Can you work these out from the model? Positions are in its coordinate system, mm. A direction names the side the tool comes from. Coordinates: 2 decimals unless noted, no trailing zeros. Order: outer loops, then holes, each group sorted by start corner. A loop starts at its lowest first (then second) coordinate and runs counter-clockwise, first axis right, second up. Notation, with made-up numbers: (22.25, 64) -> (43.25, 64) arc R31 cw to (43.25, 98) -> close; hole circle Ø1 at (-12, 39.5). An arc over 180 degrees is marked (long way). Answer in a Markdown table with one row per item.
```python
from build123d import *

# Parameters (mm, degrees)
EXTRUDE_1_DEPTH       = 2.5
SKETCH_1_3_W          = 21.9
SKETCH_1_3_H          = 3
EXTRUDE_2_DEPTH       = 0.5
SKETCH_2_R            = 1
CUT_EXTRUDE_1_DEPTH   = 34.660057049
SKETCH_3_W            = 21.9
SKETCH_3_H            = 3
CUT_EXTRUDE_2_DEPTH   = 1.5
SKETCH_4_W            = 39.2
SKETCH_4_H            = 52.23
EXTRUDE_3_DEPTH       = 1
CUT_EXTRUDE_START     = -1
CUT_EXTRUDE_3_DEPTH   = 1
FILLET_1_R            = 4
CUT_EXTRUDE_1_2_DEPTH = 1


with BuildPart() as part:
    # Sketch 1 → Extrude 1 (new body)
    with BuildSketch(Plane(origin=(0, 0, 0), x_dir=(1, 0, 0), z_dir=(0, 1, 0))):
        with BuildLine():
            ThreePointArc((13.158319986, 21.726795167), (16.799919909, 20.21839509), (18.308319986, 16.576795167))
            Line((18.308319986, 16.576795167), (18.308319986, 26.726795167))
            Line((18.308319986, 26.726795167), (13.158319986, 26.726795167))
            Line((13.158319986, 26.726795167), (13.158319986, 23.726795167))
            Line((13.158319986, 23.726795167), (-8.741680014, 23.726795167))
            Line((-8.741680014, 23.726795167), (-8.741680014, 26.726795167))
            Line((-8.741680014, 26.726795167), (-13.891680014, 26.726795167))
            Line((-13.891680014, 26.726795167), (-13.891680014, 16.576795167))
            ThreePointArc((-13.891680014, 16.576795167), (-12.383279937, 20.21839509), (-8.741680014, 21.726795167))
            Line((-8.741680014, 21.726795167), (13.158319986, 21.726795167))
        make_face()
        Polygon((-13.891680014, -22.503204833), (-13.891680014, -12.353204833), (-13.891680014, 16.576795167), (-13.891680014, 26.726795167), (-15.891680014, 26.726795167), (-15.891680014, -22.503204833), align=None)
        with BuildLine():
            ThreePointArc((13.158319986, -17.503204833), (16.799919909, -15.994804756), (18.308319986, -12.353204833))
            Line((18.308319986, -12.353204833), (18.308319986, -22.503204833))
            Line((18.308319986, -22.503204833), (-13.891680014, -22.503204833))
            Line((-13.891680014, -22.503204833), (-13.891680014, -12.353204833))
            ThreePointArc((-13.891680014, -12.353204833), (-12.383279937, -15.994804756), (-8.741680014, -17.503204833))
            Line((-8.741680014, -17.503204833), (13.158319986, -17.503204833))
        make_face()
        Polygon((18.308319986, 16.576795167), (18.308319986, -12.353204833), (18.308319986, -22.503204833), (20.308319986, -22.503204833), (20.308319986, 26.726795167), (18.308319986, 26.726795167), align=None)
    extrude(amount=EXTRUDE_1_DEPTH)

    # Sketch 1_3 → Extrude 2 (add)
    with BuildSketch(Plane(origin=(0, 0, 0), x_dir=(1, 0, 0), z_dir=(0, 1, 0))):
        with Locations((2.208319986, 25.226795167)):
            Rectangle(SKETCH_1_3_W, SKETCH_1_3_H)
    extrude(amount=EXTRUDE_2_DEPTH)

    # Sketch 2 → Cut-Extrude 1 (cut, through all)
    with BuildSketch(Plane.XZ):
        with Locations(Location((-11.891680014, -24.726795167, 0), (0, 0, 270))):
            Circle(SKETCH_2_R)
        with Locations(Location((-11.891680014, 20.503204833, 0), (0, 0, 270))):
            Circle(SKETCH_2_R)
        with Locations(Location((16.308319986, 20.503204833, 0), (0, 0, 270))):
            Circle(SKETCH_2_R)
        with Locations(Location((16.308319986, -24.726795167, 0), (0, 0, 270))):
            Circle(SKETCH_2_R)
    extrude(amount=-CUT_EXTRUDE_1_DEPTH, mode=Mode.SUBTRACT)

    # Sketch 3 → Cut-Extrude 2 (cut)
    with BuildSketch(Plane(origin=(0, 2.5, 0), x_dir=(1, 0, 0), z_dir=(0, 1, 0))):
        with Locations((2.208319986, -19.003204833)):
            Rectangle(SKETCH_3_W, SKETCH_3_H)
    extrude(amount=-CUT_EXTRUDE_2_DEPTH, mode=Mode.SUBTRACT)

    # Sketch 4 → Extrude 3 (add)
    with BuildSketch(Plane.XZ):
        with Locations((2.208319986, -2.111795167)):
            Rectangle(SKETCH_4_W, SKETCH_4_H)
    extrude(amount=EXTRUDE_3_DEPTH)

    # Sketch 5 → Cut-Extrude 3 (cut)
    with BuildSketch(Plane(origin=(0, 0, 0), x_dir=(1, 0, 0), z_dir=(0, 1, 0)).offset(CUT_EXTRUDE_START)):
        with BuildLine():
            Line((18.308319986, -12.353204833), (18.308319986, 16.576795167))
            ThreePointArc((18.308319986, 16.576795167), (16.799919909, 20.21839509), (13.158319986, 21.726795167))
            Line((13.158319986, 21.726795167), (-8.741680014, 21.726795167))
            ThreePointArc((-8.741680014, 21.726795167), (-12.383279937, 20.21839509), (-13.891680014, 16.576795167))
            Line((-13.891680014, 16.576795167), (-13.891680014, -12.353204833))
            ThreePointArc((-13.891680014, -12.353204833), (-12.383279937, -15.994804756), (-8.741680014, -17.503204833))
            Line((-8.741680014, -17.503204833), (13.158319986, -17.503204833))
            ThreePointArc((13.158319986, -17.503204833), (16.799919909, -15.994804756), (18.308319986, -12.353204833))
        make_face()
    extrude(amount=CUT_EXTRUDE_3_DEPTH, mode=Mode.SUBTRACT)

    # Fillet 1
    fillet_1_edges = [part.edges().sort_by_distance(p)[0] for p in [
        (-15.891680014, 1.25, 22.503204833),
        (-15.891680014, 1.25, -26.726795167),
        (20.308319986, 1.25, -26.726795167),
        (20.308319986, 1.25, 22.503204833),
    ]]
    fillet(fillet_1_edges, radius=FILLET_1_R)

    # Sketch 5_2 → Cut-Extrude 1 2 (cut)
    with BuildSketch(Plane(origin=(0, 0, 0), x_dir=(1, 0, 0), z_dir=(0, 1, 0)).offset(CUT_EXTRUDE_START)):
        with BuildLine():
            Line((-8.741680014, -18.003204833), (13.158319986, -18.003204833))
            ThreePointArc((13.158319986, -18.003204833), (17.153473299, -16.348358147), (18.808319986, -12.353204833))
            Line((18.808319986, -12.353204833), (18.808319986, 16.576795167))
            ThreePointArc((18.808319986, 16.576795167), (17.153473299, 20.571948481), (13.158319986, 22.226795167))
            Line((13.158319986, 22.226795167), (-8.741680014, 22.226795167))
            ThreePointArc((-8.741680014, 22.226795167), (-12.736833328, 20.571948481), (-14.391680014, 16.576795167))
            Line((-14.391680014, 16.576795167), (-14.391680014, -12.353204833))
            ThreePointArc((-14.391680014, -12.353204833), (-12.736833328, -16.348358147), (-8.741680014, -18.003204833))
        make_face()
        with BuildLine():
            Line((-8.741680014, -17.503204833), (13.158319986, -17.503204833))
            ThreePointArc((13.158319986, -17.503204833), (16.799919909, -15.994804756), (18.308319986, -12.353204833))
            Line((18.308319986, -12.353204833), (18.308319986, 16.576795167))
            ThreePointArc((18.308319986, 16.576795167), (16.799919909, 20.21839509), (13.158319986, 21.726795167))
            Line((13.158319986, 21.726795167), (-8.741680014, 21.726795167))
            ThreePointArc((-8.741680014, 21.726795167), (-12.383279937, 20.21839509), (-13.891680014, 16.576795167))
            Line((-13.891680014, 16.576795167), (-13.891680014, -12.353204833))
            ThreePointArc((-13.891680014, -12.353204833), (-12.383279937, -15.994804756), (-8.741680014, -17.503204833))
        make_face(mode=Mode.SUBTRACT)
    extrude(amount=CUT_EXTRUDE_1_2_DEPTH, mode=Mode.SUBTRACT)


solid = part.part
```
(1) Suppose I cut it at C-C (z = 14). Please give me the cut outline in (x, y).
Response values:
| item | result |
|---|---|
| outline | (-17.39, -1) -> (-14.15, -1) -> (-14.15, 0) -> (-13.62, 0) -> (-13.62, 2.5) -> (-15.89, 2.5) -> (-15.89, 0) -> (-17.39, 0) -> close; (18.04, 0) -> (18.56, 0) -> (18.56, -1) -> (21.81, -1) -> (21.81, 0) -> (20.31, 0) -> (20.31, 2.5) -> (18.04, 2.5) -> close |
(2) On a 3-axis mill with a long thin cutter (end or side, diameter ignored), from which of +Z, -Z, +X, -X, +Y, -Y can I reach the whole of each face in a straight line? I mean faces 5 (the cylindrical face through (-12.69, -0.51, -20.62)), 6 (the cylindrical face through (-12.423, 1.232, 15.955)), 7 (the flat face through (-12, 0, 21)). Say none if no direction works.
Response values:
| item | result |
|---|---|
| face 5 | -Y |
| face 6 | +Y, -Y |
| face 7 | +Y |
(3) I need wall thicknesses on line 1 (Z direction, x = -9, y = 0.9); line 2 (Z direction, x = -9, y = -0.15); line 3 (X direction, y = -0.8, z = -11). Which ranges of each line are inside material? Lowest first, please. Write a range as [from, to].
Response values:
| item | result |
|---|---|
| line 1 | [-26.73, -21.72], [17.5, 22.5] |
| line 2 | [-28.23, -22.22], [18, 24] |
| line 3 | [-17.39, -14.39], [18.81, 21.81] |
(4) Suppose I cut it at B-B (z = -9). Please give me the cut outline in (x, y).
Response values:
| item | result |
|---|---|
| outline | (-17.39, -1) -> (-14.39, -1) -> (-14.39, 0) -> (-13.89, 0) -> (-13.89, 2.5) -> (-15.89, 2.5) -> (-15.89, 0) -> (-17.39, 0) -> close; (18.31, 0) -> (18.81, 0) -> (18.81, -1) -> (21.81, -1) -> (21.81, 0) -> (20.31, 0) -> (20.31, 2.5) -> (18.31, 2.5) -> close |
(5) Suppose I cut it at A-A (x = 5.5). Please give me the cut outline in (y, z), and give its area (3 significant figures).
Response values:
| item | result |
|---|---|
| outline | (-1, -28.23) -> (0, -28.23) -> (0, -26.73) -> (0.5, -26.73) -> (0.5, -23.73) -> (2.5, -23.73) -> (2.5, -21.73) -> (0, -21.73) -> (0, -22.23) -> (-1, -22.23) -> close; (-1, 18) -> (0, 18) -> (0, 17.5) -> (1, 17.5) -> (1, 20.5) -> (2.5, 20.5) -> (2.5, 22.5) -> (0, 22.5) -> (0, 24) -> (-1, 24) -> close |
| area | 26.5 mm2 |
(6) We'd pull the mould along X, two halves only. Please class faces 1 (the flat face through (2, 1, -21.727)), 2 (the cylindrical face through (-14.75, 1.27, 21.3)), 3 (the flat face through (2.1, -0.5, 18.003)), 4 (the cylindrical face through (19.11, 1.27, 21.36)): +X half, -X half, draft (parallel to the pull), parting line (faces both ways), or undercut.
Response values:
| item | result |
|---|---|
| face 1 | undercut |
| face 2 | -X half |
| face 3 | undercut |
| face 4 | +X half |
(7) Will these pins go through, and if not, where does the flat tip stop? pin 1 Ø1.6 at (x, z) = (-11.89, 20.5) entering from +Y; pin 2 Ø1.2 at (x, y) = (-1, 1) entering from +Z; pin 3 Ø0.6 at (y, z) = (1.5, -25.5) entering from -X; pin 4 Ø12 at (x, z) = (12, 1) entering from -Y.
Response values:
| item | result |
|---|---|
| pin 1 | y = 0 |
| pin 2 | z = 22.5 |
| pin 3 | x = -15.04 |
| pin 4 | through |
